from build123d import *

# Parameters (mm, degrees)
SKETCH_1_R      = 9.5
SKETCH_1_R_2    = 8.6
EXTRUDE_2_DEPTH = 1
SKETCH_1_4_R    = 8.6
EXTRUDE_4_DEPTH = 10.5


with BuildPart() as part:
    # 草图1 → 凸台-拉伸2 (new body)
    with BuildSketch(Plane(origin=(0, 0, 0), x_dir=(1, 0, 0), z_dir=(0, 1, 0))):
        Circle(SKETCH_1_R)
        Circle(SKETCH_1_R_2, mode=Mode.SUBTRACT)
    extrude(amount=EXTRUDE_2_DEPTH)

    # 草图1<4> → 凸台-拉伸4 (add)
    with BuildSketch(Plane(origin=(0, 0, 0), x_dir=(1, 0, 0), z_dir=(0, 1, 0))):
        Circle(SKETCH_1_4_R)
        with BuildLine():
            ThreePointArc((-4.257529302, 1.319914676), (-3.22106843, 0.640114314), (-2.442480608, -0.324344434))
            Line((-2.442480608, -0.324344434), (-1.502130823, -1.953078038))
            ThreePointArc((-1.502130823, -1.953078038), (-1.056178958, -3.109584244), (-0.98568501, -4.347085871))
            Line((-0.98568501, -4.347085871), (-1.222344473, -6.737988124))
            ThreePointArc((-1.222344473, -6.737988124), (-1.673731111, -7.478733269), (-2.534264377, -7.58798419))
            ThreePointArc((-2.534264377, -7.58798419), (-4, -6.92820323), (-5.304254883, -5.988729426))
            ThreePointArc((-5.304254883, -5.988729426), (-6.92820323, -4), (-7.838519261, -1.599254764))
            ThreePointArc((-7.838519261, -1.599254764), (-8, 0), (-7.838519261, 1.599254764))
            ThreePointArc((-7.838519261, 1.599254764), (-7.313638554, 2.289872973), (-6.446441123, 2.310412696))
            Line((-6.446441123, 2.310412696), (-4.257529302, 1.319914676))
        make_face(mode=Mode.SUBTRACT)
        with BuildLine():
            ThreePointArc((2.442480608, -0.324344434), (3.22106843, 0.640114314), (4.257529302, 1.319914676))
            Line((4.257529302, 1.319914676), (6.446441123, 2.310412696))
            ThreePointArc((6.446441123, 2.310412696), (7.313638554, 2.289872973), (7.838519261, 1.599254764))
            ThreePointArc((7.838519261, 1.599254764), (8, 0), (7.838519261, -1.599254764))
            ThreePointArc((7.838519261, -1.599254764), (6.92820323, -4), (5.304254883, -5.988729426))
            ThreePointArc((5.304254883, -5.988729426), (4, -6.92820323), (2.534264377, -7.58798419))
            ThreePointArc((2.534264377, -7.58798419), (1.673731111, -7.478733269), (1.222344473, -6.737988124))
            Line((1.222344473, -6.737988124), (0.98568501, -4.347085871))
            ThreePointArc((0.98568501, -4.347085871), (1.056178958, -3.109584244), (1.502130823, -1.953078038))
            Line((1.502130823, -1.953078038), (2.442480608, -0.324344434))
        make_face(mode=Mode.SUBTRACT)
        with BuildLine():
            Line((5.22409665, 4.427575428), (3.271844291, 3.027171194))
            ThreePointArc((3.271844291, 3.027171194), (2.164889472, 2.469469931), (0.940349784, 2.277422472))
            Line((0.940349784, 2.277422472), (-0.940349784, 2.277422472))
            ThreePointArc((-0.940349784, 2.277422472), (-2.164889472, 2.469469931), (-3.271844291, 3.027171194))
            Line((-3.271844291, 3.027171194), (-5.22409665, 4.427575428))
            ThreePointArc((-5.22409665, 4.427575428), (-5.639907443, 5.188860296), (-5.304254883, 5.988729426))
            ThreePointArc((-5.304254883, 5.988729426), (-4, 6.92820323), (-2.534264377, 7.58798419))
            ThreePointArc((-2.534264377, 7.58798419), (0, 8), (2.534264377, 7.58798419))
            ThreePointArc((2.534264377, 7.58798419), (4, 6.92820323), (5.304254883, 5.988729426))
            ThreePointArc((5.304254883, 5.988729426), (5.639907443, 5.188860296), (5.22409665, 4.427575428))
        make_face(mode=Mode.SUBTRACT)
        with BuildLine():
            Line((1.229837388, -1.1), (-1.229837388, -1.1))
            ThreePointArc((-1.229837388, -1.1), (0, 1.65), (1.229837388, -1.1))
        make_face(mode=Mode.SUBTRACT)
    extrude(amount=EXTRUDE_4_DEPTH)


solid = part.part
Verification items for the finished model (mm, model axes). A direction names the side the tool comes from. Give positions to 0.01 mm unless a question says otherwise; leave off trailing zeros. Loops run counter-clockwise (first coordinate to the right, second up) from the corner with the lowest first, then second, coordinate; pieces in that order, holes last. Notation, with made-up numbers: (89, 55.25) - (102, 55.25) arc R18 ccw to (102, 64.25) - close; hole circle Ø2 at (42.25, 4). An arc over 180 degrees is marked (long way). Write item = value, one per line. Start each with the question number.
Q1. Cross-section at B-B, the plane y = 1.75. Enter the section's corners in (x, z).
Q2. Depth check by flat-ended pin: P1, Ø1.5, axis at x = 0, y = 4, coming from the -Z side; P2, Ø1, axis at x = -2.5, z = 5.5, coming from the +Y side; P3, Ø3, axis at x = 2, y = 8.5, coming from the +Z side; P4, Ø4, axis at x = 6, y = 7.5, coming from the +Z side. Enter the tip coordinate at first touch or a pass-through.
Q3. Cross-section at C-C, the plane z = 0.75. Enter the section's corners in (x, y).
Q4. Cross-section at D-D, the plane z = 8. Enter the section's corners in (x, y).
Q5. Cross-section at A-A, the plane x = 0. Enter the section's corners in (y, z).
Q6. Mould release check, pull along X, two halves, no side actions. Record for faces 1 (the face through (4.38, 0.49, 8.43)), 2 (the face through (-2.148, 5.176, -2.464)), 3 (the face through (-2.2, 1, -8.5)): released by +X, released by -X, zero draft, split by the parting line, or undercut.
Q7. Tool access check on faces 4 (the face through (-1.31, 10.5, 1.23)), 5 (the face through (1.684, 5.176, 7.485)). Record the directions out of +Z, -Z, +X, -X, +Y, -Y that give a thin tool (end or side, any length) a straight path to the whole face; none if there is none.
Q8. Thickness scan on line 1 (Z direction, x = 2.25, y = 10); line 2 (Z direction, x = -0.25, y = 3.25); line 3 (X direction, y = 4.25, z = 2.5). Record the ranges inside material, lowest first.
Answer key:
q1.outline = circle Ø17.2 at (0, 0); hole (-7.84, -1.6) arc R1 ccw to (-6.45, -2.31) - (-4.26, -1.32) arc R4 ccw to (-2.44, 0.32) - (-1.5, 1.95) arc R4 ccw to (-0.99, 4.35) - (-1.22, 6.74) arc R1 ccw to (-2.53, 7.59) arc R8 ccw to start; hole (-5.3, -5.99) arc R8 ccw to (5.3, -5.99) arc R1 ccw to (5.22, -4.43) - (3.27, -3.03) arc R4 ccw to (0.94, -2.28) - (-0.94, -2.28) arc R4 ccw to (-3.27, -3.03) - (-5.22, -4.43) arc R1 ccw to start; hole (-1.23, 1.1) arc R1.65 ccw (long way) to (1.23, 1.1) - close; hole (0.99, 4.35) arc R4 ccw to (1.5, 1.95) - (2.44, 0.32) arc R4 ccw to (4.26, -1.32) - (6.45, -2.31) arc R1 ccw to (7.84, -1.6) arc R8 ccw to (2.53, 7.59) arc R1 ccw to (1.22, 6.74) - close
q2.P1 = -8.6
q2.P2 = through
q2.P3 = 8.59
q2.P4 = 7.61
q3.outline = (-9.47, 0) - (-7.96, 0) - (-7.96, 10.5) - (-8.57, 10.5) - (-8.57, 1) - (-9.47, 1) - close; (-2.2, 0) - (-1.47, 0) - (-1.47, 10.5) - (-2.2, 10.5) - close; (1.47, 0) - (2.2, 0) - (2.2, 10.5) - (1.47, 10.5) - close; (7.96, 0) - (9.47, 0) - (9.47, 1) - (8.57, 1) - (8.57, 10.5) - (7.96, 10.5) - close
q4.outline = (-5.12, 0) - (5.12, 0) - (5.12, 1) - (3.16, 1) - (3.16, 10.5) - (-3.16, 10.5) - (-3.16, 1) - (-5.12, 1) - close
q5.outline = (0, -9.5) - (1, -9.5) - (1, -8.6) - (10.5, -8.6) - (10.5, -8) - (0, -8) - close; (0, -2.28) - (10.5, -2.28) - (10.5, -1.65) - (0, -1.65) - close; (0, 1.1) - (10.5, 1.1) - (10.5, 8.6) - (1, 8.6) - (1, 9.5) - (0, 9.5) - close
q6.face_1 = split by the parting line
q6.face_2 = undercut
q6.face_3 = zero draft
q7.face_4 = +Z, -Z, +X, -X, +Y
q7.face_5 = +Y, -Y
q8.line_1 = -8.3 to -7.68, -2.5 to 0.66, 7.64 to 8.3
q8.line_2 = -8.6 to -8, -2.28 to -1.63, 1.1 to 8.6
q8.line_3 = -8.23 to -7.6, -1.24 to 1.24, 7.6 to 8.23
